Build history of the part. All positions in model axes, mm. Face numbers are marked on the shaded views. Round coordinates to 2 decimals unless told otherwise and drop trailing zeros. Write each loop counter-clockwise with the first axis right and the second up, starting at its lowest first coordinate (ties: lowest second). Pieces come first, ordered by that corner, then holes. Notation, with made-up numbers: M -33,1.25 L 14,1.25 A20 ccw 14,40.25 Z; hole C 36,-35.5 d11. An arc over 180 degrees is marked long. Write item = value, one per line. Start each with the question number.
Q1. Band-saw the part on C-C on z = -66. Write the cut outline in (x, y).
Q2. Band-saw the part on A-A on y = 10.25. Write the cut outline in (x, z), plus the area to 3 significant figures.
Q3. Drop flat-ended pins along their axis: P1, Ø15.5, axis at x = 49, z = -29.5, coming from the +Y side; P2, Ø3, axis at y = 7, z = 7.5, coming from the -X side; P3, Ø7, axis at x = 65.5, y = 9, coming from the -Z side. Give the stop position or say it passes through.
Q4. Band-saw the part on D-D on z = -49. Write the cut outline in (x, y).
Q5. Band-saw the part on B-B on x = 67.5. Write the cut outline in (y, z).
Q6. Pull direction Z, two halves, no side cores. Call the marked faces 1 and 2: released by +Z, released by -Z, zero draft, split by the parting line, or undercut.
Q7. Probe L1, parallel to X at y = 6.75, z = -9.5; L2, parallel to Z at x = 67.5, y = 9.5; L3, parallel to Z at x = 22, y = 2.75. List the from-to ranges inside material, lowest first.
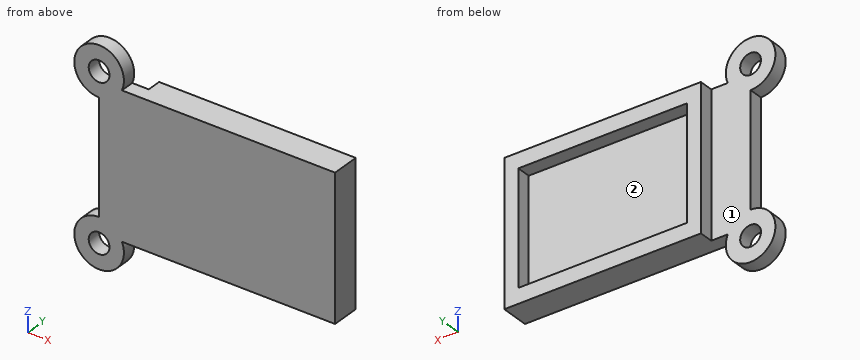
Autodesk Inventor part; units mm, degrees
ref_plane "YZ Plane" through (0, 0, 0) normal (1, 0, 0) x (0, 1, 0)
ref_plane "XZ Plane" through (0, 0, 0) normal (0, 1, 0) x (-1, 0, 0)
ref_plane "XY Plane" through (0, 0, 0) normal (0, 0, 1) x (1, 0, 0)
sketch "Sketch1" plane through (0, 0, 0) normal (0, 1, 0) x (-1, 0, 0)
  circle A0 centre (-2.8575, -62.5475) radius 4.699
  circle A1 centre (-2.8575, 11.1125) radius 4.699
  arc A2 (-2.8575, -0.1128) -> (-13.1816, 6.7056) centre (-2.8575, 11.1125) ccw
  arc A3 (-13.1816, -58.1406) -> (-2.8575, -51.3222) centre (-2.8575, -62.5475) ccw
  line L0 (-13.1816, 6.7056) -> (-109.5375, 6.7056)
  line L1 (-109.5375, 6.7056) -> (-109.5375, -58.1406)
  line L2 (-109.5375, -58.1406) -> (-13.1816, -58.1406)
  line L3 (-2.8575, -51.3222) -> (-2.8575, -0.1128)
  line L4 (-2.8575, -0.1128) -> (-2.8575, -51.3222)
  line L5 (-103.1875, -51.3222) -> (-26.9875, -51.3222)
  line L6 (-26.9875, -51.3222) -> (-26.9875, -0.1128)
  line L7 (-26.9875, -0.1128) -> (-103.1875, -0.1128)
  line L8 (-103.1875, -0.1128) -> (-103.1875, -51.3222)
  line L9 (-20.6375, 6.7056) -> (-20.6375, -58.1406)
  point P0 (0, 0)
  dimension "d1" = 9.398
  dimension "d2" = 9.398
  dimension "d4" = 6.35
extrude "Extrusion1" add sketch "Sketch1" along normal blind 6.35 contours L3 A3 L2 L9 L0 A2 | L9 L2 L1 L0 | L8 L7 L6 L5
sketch "Sketch2" plane through (0, 6.35, 0) normal (0, 1, 0) x (1, 0, 0)
  line L0 (26.9875, 0.1128) -> (103.1875, 0.1128)
  line L1 (103.1875, 0.1128) -> (103.1875, 51.3222)
  line L2 (103.1875, 51.3222) -> (26.9875, 51.3222)
  line L3 (26.9875, 51.3222) -> (26.9875, 0.1128)
  line L4 (13.1816, -6.7056) -> (109.5375, -6.7056)
  line L5 (20.6375, -6.7056) -> (20.6375, 58.7375)
  line L6 (109.5375, 58.1406) -> (13.1816, 58.1406)
  line L7 (20.6375, -6.7056) -> (109.5375, -6.7056)
  line L8 (109.5375, -6.7056) -> (109.5375, 58.1406)
  line L9 (109.5375, 58.1406) -> (20.6375, 58.1406)
  line L10 (20.6375, 58.1406) -> (20.6375, -6.7056)
  point P0 (0, 0)
  dimension "d7" = 6.35
extrude "Extrusion2" add sketch "Sketch2" along normal blind 6.35
properties part number "ignition mount"
Conclusion:
q1.outline = M -7.82,0 L -0.33,0 L -0.33,6.35 L -7.82,6.35 Z; M 6.05,0 L 13.54,0 L 13.54,6.35 L 6.05,6.35 Z
q2.outline = M 20.64,-58.14 L 109.54,-58.14 L 109.54,6.71 L 20.64,6.71 Z; hole M 26.99,-51.32 L 103.19,-51.32 L 103.19,-0.11 L 26.99,-0.11 Z
q2.area = 1,860 mm^2
q3.P1 = 6.35
q3.P2 = -8.14
q3.P3 = -58.14
q4.outline = M 2.86,0 L 109.54,0 L 109.54,12.7 L 103.19,12.7 L 103.19,6.35 L 26.99,6.35 L 26.99,12.7 L 20.64,12.7 L 20.64,6.35 L 2.86,6.35 Z
q5.outline = M 0,-58.14 L 12.7,-58.14 L 12.7,-51.32 L 6.35,-51.32 L 6.35,-0.11 L 12.7,-0.11 L 12.7,6.71 L 0,6.71 Z
q6.face_1 = zero draft
q6.face_2 = undercut
q7.L1 = 20.64 to 26.99, 103.19 to 109.54
q7.L2 = -58.14 to -51.32, -0.11 to 6.71
q7.L3 = -58.14 to 6.71
